Work out the finished part from the listing and answer in its coordinate system (mm). Round coordinates to 2 decimals unless told otherwise and drop trailing zeros. Order: outer loops, then holes, each group sorted by start corner. A loop starts at its lowest first (then second) coordinate and runs counter-clockwise, first axis right, second up. Notation, with made-up numbers: M 41.5,61 L 79.5,61 A15 cw 79.5,79 Z; hole C 1,82 d4. An arc over 180 degrees is marked long. Answer as a JSON object with one key per item and string values. Group by question number.
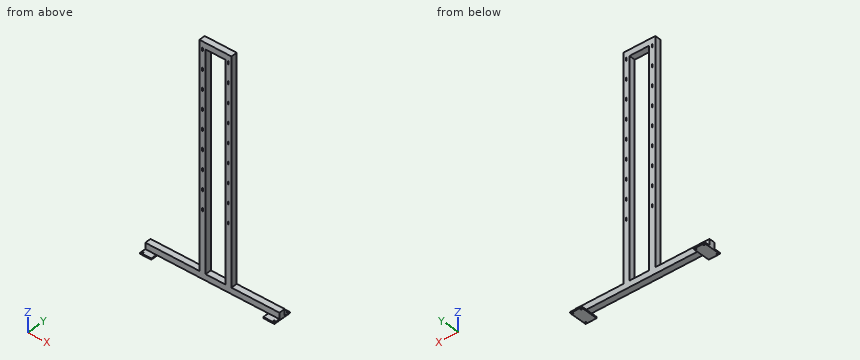
from build123d import *

# Parameters (mm, degrees)
F0_W      = 90
F0_H      = 145
F1_DEPTH  = 10
F3_D      = 13.2
F4_W      = 90
F4_H      = 50
F5_DEPTH  = 50
F6_W      = 50
F6_H      = 50
F7_DEPTH  = 1000
F8_W      = 90
F8_H      = 145
F9_DEPTH  = 10
F11_D     = 13.2
F12_W     = 50
F12_H     = 50
F13_DEPTH = 1790
F14_W     = 260
F14_H     = 50
F15_DEPTH = 50
F16_W     = 6
F16_H     = 25.2000307604
F17_DEPTH = 97.501


with BuildPart() as f1:
    # F0 (on Top) → F1 (new body)
    with BuildSketch(Plane.XY):
        Rectangle(F0_W, F0_H)
    extrude(amount=F1_DEPTH)

    # F3 (through all)
    with Locations(Plane(origin=(0, 0, 0), x_dir=(1, 0, 0), z_dir=(0, 0, -1))):
        with Locations((35, -62.5), (35, 62.5), (-35, -62.5)):
            Hole(F3_D / 2)

    # F4 (on face) → F5 (join)
    with BuildSketch(Plane.XY.offset(10)):
        Rectangle(F4_W, F4_H)
    extrude(amount=F5_DEPTH)

    # F6 (on face) → F7 (join)
    with BuildSketch(Plane(origin=(-45, 0, 0), x_dir=(0, -1, 0), z_dir=(-1, 0, 0))):
        with Locations((0, 35)):
            Rectangle(F6_W, F6_H)
    extrude(amount=F7_DEPTH)

    # F8 (on face) → F9 (join)
    with BuildSketch(Plane(origin=(0, 0, 10), x_dir=(1, 0, 0), z_dir=(0, 0, -1))):
        with Locations((-1000, 0)):
            Rectangle(F8_W, F8_H)
    extrude(amount=F9_DEPTH)

    # F11 (through all)
    with Locations(Plane.XY.offset(10)):
        with Locations((-965, 62.5), (-1035, -62.5), (-1035, 62.5)):
            Hole(F11_D / 2)

    # F12 (on face) → F13 (join)
    with BuildSketch(Plane.XY.offset(60)):
        with Locations((-370, 0)):
            Rectangle(F12_W, F12_H)
        with Locations((-580, 0)):
            Rectangle(F12_W, F12_H)
    extrude(amount=F13_DEPTH)

    # F14 (on face) → F15 (join)
    with BuildSketch(Plane.XY.offset(1850)):
        with Locations((-475, 0)):
            Rectangle(F14_W, F14_H)
    extrude(amount=-F15_DEPTH)

    # F16 (on face) → F17 (cut, through all)
    with BuildSketch(Plane.XZ.offset(25)):
        with Locations((-370, 547.6000153802)):
            Rectangle(F16_W, F16_H)
        with Locations((-370, 702.6000153802)):
            Rectangle(F16_W, F16_H)
        with Locations((-370, 857.6000153802)):
            Rectangle(F16_W, F16_H)
        with Locations((-370, 1012.6000153802)):
            Rectangle(F16_W, F16_H)
        with Locations((-370, 1167.6000153802)):
            Rectangle(F16_W, F16_H)
        with Locations((-370, 1322.6000153802)):
            Rectangle(F16_W, F16_H)
        with Locations((-370, 1477.6000153802)):
            Rectangle(F16_W, F16_H)
        with Locations((-370, 1632.6000153802)):
            Rectangle(F16_W, F16_H)
        with Locations((-370, 1787.6000153802)):
            Rectangle(F16_W, F16_H)
        with Locations((-580, 547.6000153802)):
            Rectangle(F16_W, F16_H)
        with Locations((-580, 702.6000153802)):
            Rectangle(F16_W, F16_H)
        with Locations((-580, 857.6000153802)):
            Rectangle(F16_W, F16_H)
        with Locations((-580, 1012.6000153802)):
            Rectangle(F16_W, F16_H)
        with Locations((-580, 1167.6000153802)):
            Rectangle(F16_W, F16_H)
        with Locations((-580, 1322.6000153802)):
            Rectangle(F16_W, F16_H)
        with Locations((-580, 1477.6000153802)):
            Rectangle(F16_W, F16_H)
        with Locations((-580, 1632.6000153802)):
            Rectangle(F16_W, F16_H)
        with Locations((-580, 1787.6000153802)):
            Rectangle(F16_W, F16_H)
    extrude(amount=-F17_DEPTH, mode=Mode.SUBTRACT)


solid = f1.part
Item 1: Each of these flat-tipped pins is pushed along its axis until it touches: pin 1 (5 mm diameter, centred on x = -370.5, y = -10.5, fed in from -Z); pin 2 (2 mm diameter, centred on y = 3, z = 1385.5, fed in from +X); pin 3 (2 mm diameter, centred on x = -572.5, z = 1285.5, fed in from -Y). Where does it stop, or does it pass through?
Item 2: Find section C-C (x = -912). Give the vertices of the cut face in (y, z).
Item 3: Find section B-B (z = 229.5). Give the vertices of the cut face in (x, y).
Item 4: Find section A-A (x = -470). Give the vertices of the cut face in (y, z), and give its area (3 significant figures).
Item 5: Consider L1, parallel to Y at x = -1035, z = 5.5; L2, parallel to X at y = 14.5, z = 324; L3, parallel to Y at x = -35, z = 5.5. Determine where each line is inside the solid, lowest interval first.
Responses:
{
 "1": {"pin 1": "stops at z = 10", "pin 2": "stops at x = -345", "pin 3": "stops at y = -25"},
 "2": {"outline": "M -25,10 L 25,10 L 25,60 L -25,60 Z"},
 "3": {"outline": "M -605,-25 L -555,-25 L -555,25 L -605,25 Z; M -395,-25 L -345,-25 L -345,25 L -395,25 Z"},
 "4": {"outline": "M -25,10 L 25,10 L 25,60 L -25,60 Z; M -25,1800 L 25,1800 L 25,1850 L -25,1850 Z", "area": "5,000 mm^2"},
 "5": {"L1": "y = -72.5 to -69.1, -55.9 to 55.9, 69.1 to 72.5", "L2": "x = -605 to -555, -395 to -345", "L3": "y = -72.5 to 55.9, 69.1 to 72.5"}
}
